from build123d import *

# Parameters (mm, degrees)
SKETCH1_W                                           = 58
SKETCH1_H                                           = 28
BOSS_EXTRUDE1_DEPTH                                 = 7
CBORE_FOR_M4_HEX_SOCKET_HEAD_CAP_SCREW1_D           = 4.3
CBORE_FOR_M4_HEX_SOCKET_HEAD_CAP_SCREW1_CBORE_D     = 8
CBORE_FOR_M4_HEX_SOCKET_HEAD_CAP_SCREW1_CBORE_DEPTH = 4.4


with BuildPart() as part:
    # Sketch1 → Boss-Extrude1 (new, symmetric)
    with BuildSketch(Plane.XY):
        Rectangle(SKETCH1_W, SKETCH1_H)
    extrude(amount=BOSS_EXTRUDE1_DEPTH, both=True)

    # CBORE for M4 Hex Socket Head Cap Screw1 (through all)
    with Locations(Plane.XY.offset(7)):
        with Locations((-11, 7.6), (11, 7.6)):
            CounterBoreHole(CBORE_FOR_M4_HEX_SOCKET_HEAD_CAP_SCREW1_D / 2, CBORE_FOR_M4_HEX_SOCKET_HEAD_CAP_SCREW1_CBORE_D / 2, CBORE_FOR_M4_HEX_SOCKET_HEAD_CAP_SCREW1_CBORE_DEPTH)


solid = part.part
Geometry: final body of the model. Coordinates: model frame, mm. A direction names the side the tool comes from. Coordinates: 2 decimals unless noted, no trailing zeros. Order: outer loops, then holes, each group sorted by start corner. A loop starts at its lowest first (then second) coordinate and runs counter-clockwise, first axis right, second up.
1) Draft query along X for faces 1 (the flat face through (-29, 0, 0)), 2 (the cylindrical face through (10.01, 5.69, -2.27)), 3 (the flat face through (0, -14, 0)). Return one class per face: released by +X, released by -X, zero draft, split by the parting line, or undercut.
Result sheet:
face 1: released by -X
face 2: undercut
face 3: zero draft
2) Section D-D (y = 4.5). Return loops of the section in (x, z).
Result sheet:
outline: (-29, -7) - (29, -7) - (29, 7) - (13.53, 7) - (13.53, 2.6) - (8.47, 2.6) - (8.47, 7) - (-8.47, 7) - (-8.47, 2.6) - (-13.53, 2.6) - (-13.53, 7) - (-29, 7) - close
3) First-contact query: P1, Ø4, axis at x = 11, y = 7.6, coming from the +Z side; P2, Ø6.5, axis at x = -11, y = 7.6, coming from the +Z side. Flat tips, straight axial feed; report the tip coordinate or a pass-through.
Result sheet:
P1: passes through
P2: stops at z = 2.6
4) Ray query, probe 1 along Y at (x, z) = (-11, 4.7); probe 2 along Y at (x, z) = (11, -0.25); probe 3 along Z at (x, y) = (9, 10.5). Return the intervals inside material, ascending.
Result sheet:
probe 1: y = -14 to 3.6, 11.6 to 14
probe 2: y = -14 to 5.45, 9.75 to 14
probe 3: z = -7 to 2.6
5) Section A-A (x = 11). Return loops of the section in (y, z).
Result sheet:
outline: (-14, -7) - (5.45, -7) - (5.45, 2.6) - (3.6, 2.6) - (3.6, 7) - (-14, 7) - close; (9.75, -7) - (14, -7) - (14, 7) - (11.6, 7) - (11.6, 2.6) - (9.75, 2.6) - close
6) Section C-C (z = 6). Return loops of the section in (x, y), then the cut area to 3 significant figures.
Result sheet:
outline: (-29, -14) - (29, -14) - (29, 14) - (-29, 14) - close; hole circle Ø8 at (-11, 7.6); hole circle Ø8 at (11, 7.6)
area: 1,520 mm2
7) Set-up query: faces 4 (the cylindrical face through (7.004, 7.776, 4.831)), 5 (the flat face through (29, 0, 0)). Return all of +Z, -Z, +X, -X, +Y, -Y with unobstructed straight access to the full face (end or side cutting, diameter ignored); none if empty.
Result sheet:
face 4: +Z
face 5: +Z, -Z, +X, +Y, -Y
8) Section B-B (y = 7.6). Return loops of the section in (x, z), then the cut area to 3 significant figures.
Result sheet:
outline: (-29, -7) - (-13.15, -7) - (-13.15, 2.6) - (-15, 2.6) - (-15, 7) - (-29, 7) - close; (-8.85, -7) - (8.85, -7) - (8.85, 2.6) - (7, 2.6) - (7, 7) - (-7, 7) - (-7, 2.6) - (-8.85, 2.6) - close; (13.15, -7) - (29, -7) - (29, 7) - (15, 7) - (15, 2.6) - (13.15, 2.6) - close
area: 659 mm2
